Design review of the part built by this model. Coordinates are the model's own, in mm. A direction names the side the tool comes from. Give positions to 0.01 mm unless a question says otherwise; leave off trailing zeros. Order: outer loops, then holes, each group sorted by start corner. A loop starts at its lowest first (then second) coordinate and runs counter-clockwise, first axis right, second up. Notation, with made-up numbers: (75, 72.5) -> (120, 72.5) arc R22 cw to (120, 95.5) -> close; hole circle Ø1 at (67.25, -0.75). An arc over 180 degrees is marked (long way). One line per item, written item: value.
from build123d import *

# Parameters (mm, degrees)
EXTRUDE_1_DEPTH = 10
SKETCH_2_R      = 1
EXTRUDE_2_DEPTH = 6


with BuildPart() as part:
    # Эскиз1 → Бобышка-Вытянуть1 (new body)
    with BuildSketch(Plane(origin=(0, 0, 0), x_dir=(1, 0, 0), z_dir=(0, 1, 0))):
        Polygon((0, -2.309401077), (2, -1.154700538), (2, 1.154700538), (0, 2.309401077), (-2, 1.154700538), (-2, -1.154700538), align=None)
    extrude(amount=EXTRUDE_1_DEPTH)

    # Эскиз2 → Бобышка-Вытянуть2 (add)
    with BuildSketch(Plane(origin=(0, 10, 0), x_dir=(1, 0, 0), z_dir=(0, 1, 0))):
        with Locations(Location((0, 0, 0), (0, 0, 270))):
            Circle(SKETCH_2_R)
    extrude(amount=EXTRUDE_2_DEPTH)


solid = part.part
Item 1: Machinability: for faces 1 (the flat face through (2, 5, 0)), 2 (the cylindrical face through (-1, 13, 0)), which of the approach directions +Z, -Z, +X, -X, +Y, -Y give a long, thin tool a straight path to every point of the face, cutting with its end or side? Answer none if there is none.
Returned:
face 1: +Z, -Z, +X, +Y, -Y
face 2: +Y
Item 2: Add section A-A on z = 0. Give the boundary of the cut face in (x, y), plus the area to 3 significant figures.
Returned:
outline: (-2, 0) -> (2, 0) -> (2, 10) -> (1, 10) -> (1, 16) -> (-1, 16) -> (-1, 10) -> (-2, 10) -> close
area: 52.0 mm²
Item 3: Clearance check with flat-ended pins moving along their axes: P1, Ø1, axis at y = 11.5, z = -0.5, coming from the -X side; P2, Ø1.5, axis at x = 1.5, y = 3, coming from the +Z side; P3, Ø1.5, axis at x = -0.5, y = 8, coming from the +Z side. State where each tip first meets the part, or that it passes through.
Returned:
P1: x = -1
P2: z = 1.88
P3: z = 2.31
Item 4: To check wall thickness, follow line 1 along Y through (x, z) = (0.55, 1.75); line 2 along Z through (x, y) = (-0.05, 12.75); line 3 along Z through (x, y) = (-0.9, 14.5). State the ranges of each line that lie inside material, in increasing order. Write a range as from..to.
Returned:
line 1: 0..10
line 2: -1..1
line 3: -0.44..0.44
Item 5: Add section D-D on y = 11.75. Give the boundary of the cut face in (x, z), plus the area to 3 significant figures.
Returned:
outline: circle Ø2 at (0, 0)
area: 3.14 mm²
Item 6: Add section B-B on y = 6. Give the boundary of the cut face in (x, z).
Returned:
outline: (-2, -1.15) -> (0, -2.31) -> (2, -1.15) -> (2, 1.15) -> (0, 2.31) -> (-2, 1.15) -> close
Item 7: Add section C-C on x = -0.3. Give the boundary of the cut face in (y, z).
Returned:
outline: (0, -2.14) -> (10, -2.14) -> (10, -0.95) -> (16, -0.95) -> (16, 0.95) -> (10, 0.95) -> (10, 2.14) -> (0, 2.14) -> close
